```python
from build123d import *

# Parameters (mm, degrees)
ESQUISSE1_W             = 6
ESQUISSE1_H             = 6
BOSS_EXTRU_1_DEPTH      = 2.5
D_GAGEMENT_M21_D        = 2.4
CHANFREIN1_SIZE         = 1.5
CHANFREIN2_SIZE         = 3
CONG_3_R                = 0.8
ENL_V_MAT_EXTRU_1_REACH = 4.5


with BuildPart() as part:
    # Esquisse1 → Boss.-Extru.1 (new body)
    with BuildSketch(Plane.XY):
        Polygon((19.677471167, 17), (48.900602827, -4.024), (67.901253291, -77.094002614), (72.595795313, -84.772627178), (62.357629227, -91.032016541), (46.285412403, -78.306693506), (46.71123265, -66.806693506), (20.391821523, -26.665834049), align=None)
        Polygon((51.023072953, -60.616622474), (28.816069815, -26.747772307), (44.278044238, -14.062058021), (55.602935243, -57.613715208), align=None, mode=Mode.SUBTRACT)
        Polygon((39.485073144, -5.706221012), (23.25, 5.973778988), (23.25, -19.026221012), align=None, mode=Mode.SUBTRACT)
        Polygon((12.25, 17), (12.25, 10), (12.25, -10), (12.25, -16), (6.25, -16), (20.391821523, -26.665834049), (19.677471167, 17), align=None)
        with Locations((9.25, -13)):
            Rectangle(ESQUISSE1_W, ESQUISSE1_H)
        Polygon((12.25, 17), (12.25, 10), (-12.25, 10), (-17.75, 10), (-17.75, 17), align=None)
    extrude(amount=BOSS_EXTRU_1_DEPTH)

    # Dégagement M21 (through all)
    with Locations(Plane.XY.offset(2.5)):
        with Locations((-13.75, 13.5), (-5.75, 13.5), (2.25, 13.5), (10.25, 13.5), (15.75, 8), (15.75, -8), (10.25, -13.5)):
            Hole(D_GAGEMENT_M21_D / 2)

    # Chanfrein1
    chanfrein1_edges = [part.edges().sort_by_distance(p)[0] for p in [
        (-17.75, 10, 1.25),
    ]]
    chamfer(chanfrein1_edges, length=CHANFREIN1_SIZE)

    # Chanfrein2
    chanfrein2_edges = [part.edges().sort_by_distance(p)[0] for p in [
        (-17.75, 17, 1.25),
    ]]
    chamfer(chanfrein2_edges, length=CHANFREIN2_SIZE)

    # Congé3
    cong_3_edges = [part.edges().sort_by_distance(p)[0] for p in [
        (12.25, -10, 1.25),
        (12.25, 10, 1.25),
    ]]
    fillet(cong_3_edges, radius=CONG_3_R)

    # Esquisse6 → Enlèv. mat.-Extru.1 (cut, up to next)
    with BuildSketch(Plane.XY.offset(2.5), mode=Mode.PRIVATE) as enl_v_mat_extru_1_sk1:
        Polygon((50.923621455, -68.720394376), (56.895885005, -65.069083914), (62.112042808, -73.600888985), (56.139779258, -77.252199447), align=None)
    enl_v_mat_extru_1_tool1 = extrude(enl_v_mat_extru_1_sk1.sketch, amount=-ENL_V_MAT_EXTRU_1_REACH, mode=Mode.PRIVATE) & part.part
    add(enl_v_mat_extru_1_tool1.solids().sort_by_distance((56.517832, -71.160642, 2.5))[0], mode=Mode.SUBTRACT)


solid = part.part
```
Read the model definition and answer for the solid it produces. Units are mm, in the model's axes. A direction names the side the tool comes from. Coordinates: 2 decimals unless noted, no trailing zeros. Loops run counter-clockwise (first coordinate to the right, second up) from the corner with the lowest first, then second, coordinate; pieces in that order, holes last.
(1) The part is cut by section D-D (y = -8). Determine the outline of the cut face in (x, z), and give its area (3 significant figures).
Solution:
outline: (12.25, 0) - (14.55, 0) - (14.55, 2.5) - (12.25, 2.5) - close; (16.95, 0) - (23.25, 0) - (23.25, 2.5) - (16.95, 2.5) - close; (36.69, 0) - (49.93, 0) - (49.93, 2.5) - (36.69, 2.5) - close
area: 54.6 mm2
(2) The part is cut by section B-B (y = 8). Determine the outline of the cut face in (x, z).
Solution:
outline: (12.25, 0) - (14.55, 0) - (14.55, 2.5) - (12.25, 2.5) - close; (16.95, 0) - (32.19, 0) - (32.19, 2.5) - (16.95, 2.5) - close
(3) The mould has two halves that part along X. Classify faces 1 (the face through (33.736, -47.017, 1.232)), 2 (the face through (36.439, -20.494, 1.232)), 3 (the face through (30.98, -24.76, 0)), 4 (the face through (40.075, -43.919, 1.232)): released by +X, released by -X, zero draft, split by the parting line, or undercut.
Solution:
face 1: released by -X
face 2: undercut
face 3: zero draft
face 4: undercut
(4) Consider line 1 along Y through (x, z) = (10.25, 1.15); line 2 along Y through (x, z) = (-13.75, 1.75); line 3 along Y through (x, z) = (34, 1). Determine where each line is inside the solid, lowest interval first.
Solution:
line 1: y = -19.02 to -14.7, -12.3 to -10, 10 to 12.3, 14.7 to 17
line 2: y = 10 to 12.3, 14.7 to 17
line 3: y = -47.42 to -34.65, -22.49 to -10.21, -1.76 to 6.7
(5) The part is cut by section A-A (x = 2.25). Determine the outline of the cut face in (y, z), and give its area (3 significant figures).
Solution:
outline: (10, 0) - (12.3, 0) - (12.3, 2.5) - (10, 2.5) - close; (14.7, 0) - (17, 0) - (17, 2.5) - (14.7, 2.5) - close
area: 11.5 mm2
(6) The part is cut by section C-C (x = 15.75). Determine the outline of the cut face in (y, z).
Solution:
outline: (-23.16, 0) - (-9.2, 0) - (-9.2, 2.5) - (-23.16, 2.5) - close; (-6.8, 0) - (6.8, 0) - (6.8, 2.5) - (-6.8, 2.5) - close; (9.2, 0) - (17, 0) - (17, 2.5) - (9.2, 2.5) - close
(7) A tool of negligible diameter and unlimited length cuts with its end or side. For faces 5 (the face through (6.25, -13, 1)), 6 (the face through (34.08, 6.64, 1.23)), 7 (the face through (53.9, -66.9, 1.3)), 8 (the face through (12.25, 0, 1)), from which of +Z, -Z, +X, -X, +Y, -Y can it reach the whole face along a straight path? Write none if from no direction.
Solution:
face 5: +Z, -Z, -X, -Y
face 6: +Z, -Z, +X, +Y
face 7: +Z, -Z
face 8: +Z, -Z, -X
(8) Flat-ended cylindrical pins translate along their axes: pin 1 Ø0.8 at (y, z) = (-10, 1) entering from +X; pin 2 Ø1.5 at (y, z) = (-61.5, 2) entering from -X; pin 3 Ø1 at (y, z) = (-45.5, 1.5) entering from -X. Find the tip coordinate at first contact, or state that the pin passes through.
Solution:
pin 1: stops at x = 50.56
pin 2: stops at x = 42.74
pin 3: stops at x = 32.41
